```python
from build123d import *

# Parameters (mm, degrees)
CROQUIS4_R              = 4
SALIENTE_EXTRUIR1_DEPTH = 1.5
SALIENTE_EXTRUIR2_DEPTH = 6.9
SALIENTE_EXTRUIR3_DEPTH = 1.5
CORTAR_EXTRUIR1_DEPTH   = 1.5
REDONDEO1_R             = 3


with BuildPart() as part:
    # Croquis4 → Saliente-Extruir1 (new body)
    with BuildSketch(Plane.XY):
        with BuildLine():
            Line((-683.531695239, 333.374182683), (-683.531695239, 346.225865369))
            ThreePointArc((-683.531695239, 346.225865369), (-682.360122363, 349.054292493), (-679.531695239, 350.225865369))
            Line((-679.531695239, 350.225865369), (-666.680012553, 350.225865369))
            ThreePointArc((-666.680012553, 350.225865369), (-665.398822158, 349.872619004), (-664.479692443, 348.912706306))
            ThreePointArc((-664.479692443, 348.912706306), (-659.289054552, 341.941594121), (-652.317942367, 336.75095623))
            ThreePointArc((-652.317942367, 336.75095623), (-651.358029669, 335.831826514), (-651.004783304, 334.550636119))
            Line((-651.004783304, 334.550636119), (-667.856465989, 317.698953434))
            ThreePointArc((-667.856465989, 317.698953434), (-669.137656384, 318.052199798), (-670.0567861, 319.012112496))
            ThreePointArc((-670.0567861, 319.012112496), (-675.247423991, 325.983224681), (-682.218536176, 331.173862573))
            ThreePointArc((-682.218536176, 331.173862573), (-683.178448874, 332.092992288), (-683.531695239, 333.374182683))
        make_face()
        with Locations((-667.975346053, 334.669516182)):
            Circle(CROQUIS4_R, mode=Mode.SUBTRACT)
        with BuildLine():
            Line((-675.753520646, 345.629671291), (-673.632200302, 343.508350947))
            ThreePointArc((-673.632200302, 343.508350947), (-673.632200302, 340.326370432), (-676.814180817, 340.326370432))
            Line((-676.814180817, 340.326370432), (-678.935501161, 342.447690776))
            ThreePointArc((-678.935501161, 342.447690776), (-678.935501161, 345.629671291), (-675.753520646, 345.629671291))
        make_face(mode=Mode.SUBTRACT)
        with BuildLine():
            Line((-669.475346053, 344.419516182), (-669.475346053, 342.419516182))
            ThreePointArc((-669.475346053, 342.419516182), (-667.975346053, 340.919516182), (-666.475346053, 342.419516182))
            Line((-666.475346053, 342.419516182), (-666.475346053, 344.419516182))
            ThreePointArc((-666.475346053, 344.419516182), (-667.975346053, 345.919516182), (-669.475346053, 344.419516182))
        make_face(mode=Mode.SUBTRACT)
        with BuildLine():
            Line((-658.225346053, 336.169516182), (-660.225346053, 336.169516182))
            ThreePointArc((-660.225346053, 336.169516182), (-661.725346053, 334.669516182), (-660.225346053, 333.169516182))
            Line((-660.225346053, 333.169516182), (-658.225346053, 333.169516182))
            ThreePointArc((-658.225346053, 333.169516182), (-656.725346053, 334.669516182), (-658.225346053, 336.169516182))
        make_face(mode=Mode.SUBTRACT)
        with BuildLine():
            Line((-666.475346053, 324.919516182), (-666.475346053, 326.919516182))
            ThreePointArc((-666.475346053, 326.919516182), (-667.975346053, 328.419516182), (-669.475346053, 326.919516182))
            Line((-669.475346053, 326.919516182), (-669.475346053, 324.919516182))
            ThreePointArc((-669.475346053, 324.919516182), (-667.975346053, 323.419516182), (-666.475346053, 324.919516182))
        make_face(mode=Mode.SUBTRACT)
        with BuildLine():
            Line((-677.725346053, 333.169516182), (-675.725346053, 333.169516182))
            ThreePointArc((-675.725346053, 333.169516182), (-674.225346053, 334.669516182), (-675.725346053, 336.169516182))
            Line((-675.725346053, 336.169516182), (-677.725346053, 336.169516182))
            ThreePointArc((-677.725346053, 336.169516182), (-679.225346053, 334.669516182), (-677.725346053, 333.169516182))
        make_face(mode=Mode.SUBTRACT)
    extrude(amount=SALIENTE_EXTRUIR1_DEPTH)

    # Croquis5 → Saliente-Extruir2 (add)
    with BuildSketch(Plane(origin=(0, 0, 0), x_dir=(-1, 0, 0), z_dir=(0, 0, -1))):
        with BuildLine():
            ThreePointArc((670.0567861, 319.012112496), (669.137656384, 318.052199798), (667.856465989, 317.698953434))
            Line((667.856465989, 317.698953434), (669.532640967, 316.022778456))
            ThreePointArc((669.532640967, 316.022778456), (670.853714641, 316.842392616), (671.817042188, 318.062639746))
            ThreePointArc((671.817042188, 318.062639746), (676.661637554, 324.569011119), (683.168008926, 329.413606484))
            ThreePointArc((683.168008926, 329.413606484), (684.895851783, 331.068039972), (685.531695239, 333.374182683))
            Line((685.531695239, 333.374182683), (685.531695239, 346.225865369))
            ThreePointArc((685.531695239, 346.225865369), (683.774335926, 350.468506056), (679.531695239, 352.225865369))
            Line((679.531695239, 352.225865369), (666.680012553, 352.225865369))
            ThreePointArc((666.680012553, 352.225865369), (664.373869842, 351.590021913), (662.719436354, 349.862179056))
            ThreePointArc((662.719436354, 349.862179056), (657.874840989, 343.355807684), (651.368469617, 338.511212318))
            ThreePointArc((651.368469617, 338.511212318), (650.148222486, 337.547884771), (649.328608326, 336.226811097))
            Line((649.328608326, 336.226811097), (651.004783304, 334.550636119))
            ThreePointArc((651.004783304, 334.550636119), (651.358029669, 335.831826514), (652.317942367, 336.75095623))
            ThreePointArc((652.317942367, 336.75095623), (659.289054552, 341.941594121), (664.479692443, 348.912706306))
            ThreePointArc((664.479692443, 348.912706306), (665.398822158, 349.872619004), (666.680012553, 350.225865369))
            Line((666.680012553, 350.225865369), (679.531695239, 350.225865369))
            ThreePointArc((679.531695239, 350.225865369), (682.360122363, 349.054292493), (683.531695239, 346.225865369))
            Line((683.531695239, 346.225865369), (683.531695239, 333.374182683))
            ThreePointArc((683.531695239, 333.374182683), (683.178448874, 332.092992288), (682.218536176, 331.173862573))
            ThreePointArc((682.218536176, 331.173862573), (675.247423991, 325.983224681), (670.0567861, 319.012112496))
        make_face()
        with BuildLine():
            ThreePointArc((678.935501161, 342.447690776), (678.935501161, 345.629671291), (675.753520646, 345.629671291))
            Line((675.753520646, 345.629671291), (673.632200302, 343.508350947))
            ThreePointArc((673.632200302, 343.508350947), (673.632200302, 340.326370432), (676.814180817, 340.326370432))
            Line((676.814180817, 340.326370432), (678.935501161, 342.447690776))
        make_face()
    extrude(amount=-SALIENTE_EXTRUIR2_DEPTH)

    # Croquis6 → Saliente-Extruir3 (add)
    with BuildSketch(Plane.XY.offset(6.9)):
        with BuildLine():
            Line((-667.856465989, 319.198953434), (-667.100243806, 318.465261145))
            Line((-667.100243806, 318.465261145), (-669.532640967, 316.022778456))
            ThreePointArc((-669.532640967, 316.022778456), (-670.853714641, 316.842392616), (-671.817042188, 318.062639746))
            ThreePointArc((-671.817042188, 318.062639746), (-676.661637554, 324.569011119), (-683.168008926, 329.413606484))
            ThreePointArc((-683.168008926, 329.413606484), (-684.895851783, 331.068039972), (-685.531695239, 333.374182683))
            Line((-685.531695239, 333.374182683), (-685.531695239, 346.225865369))
            ThreePointArc((-685.531695239, 346.225865369), (-683.774335926, 350.468506056), (-679.531695239, 352.225865369))
            Line((-679.531695239, 352.225865369), (-666.680012553, 352.225865369))
            ThreePointArc((-666.680012553, 352.225865369), (-664.373869842, 351.590021913), (-662.719436354, 349.862179056))
            ThreePointArc((-662.719436354, 349.862179056), (-657.874840989, 343.355807684), (-651.368469617, 338.511212318))
            ThreePointArc((-651.368469617, 338.511212318), (-650.148222486, 337.547884771), (-649.328608326, 336.226811097))
            Line((-649.328608326, 336.226811097), (-651.765332209, 333.790087215))
            Line((-651.765332209, 333.790087215), (-652.503991007, 334.551428417))
            ThreePointArc((-652.503991007, 334.551428417), (-652.645289552, 335.063904575), (-653.029254632, 335.431556461))
            ThreePointArc((-653.029254632, 335.431556461), (-660.349095394, 340.881501273), (-665.799494351, 348.201003883))
            ThreePointArc((-665.799494351, 348.201003883), (-666.167146237, 348.584968962), (-666.679622395, 348.726267508))
            Line((-666.679622395, 348.726267508), (-679.53130508, 348.726267508))
            ThreePointArc((-679.53130508, 348.726267508), (-681.299072033, 347.994034461), (-682.03130508, 346.226267508))
            Line((-682.03130508, 346.226267508), (-682.03130508, 333.374584822))
            ThreePointArc((-682.03130508, 333.374584822), (-681.890006535, 332.862108664), (-681.506041455, 332.494456778))
            ThreePointArc((-681.506041455, 332.494456778), (-674.186373661, 327.044286992), (-668.736203875, 319.724619198))
            ThreePointArc((-668.736203875, 319.724619198), (-668.368791902, 319.340524583), (-667.856465989, 319.198953434))
        make_face()
    extrude(amount=SALIENTE_EXTRUIR3_DEPTH)

    # Croquis7 → Cortar-Extruir1 (cut)
    with BuildSketch(Plane.XY.offset(1.5)):
        with BuildLine():
            Line((-677.725346053, 330.669516182), (-666.305624647, 319.249794777))
            Line((-666.305624647, 319.249794777), (-652.555624647, 332.999794777))
            Line((-652.555624647, 332.999794777), (-663.975346053, 344.419516182))
            ThreePointArc((-663.975346053, 344.419516182), (-667.975346053, 348.419516182), (-671.975346053, 344.419516182))
            ThreePointArc((-671.975346053, 344.419516182), (-671.975346053, 338.669516182), (-677.725346053, 338.669516182))
            ThreePointArc((-677.725346053, 338.669516182), (-681.725346053, 334.669516182), (-677.725346053, 330.669516182))
        make_face()
    extrude(amount=-CORTAR_EXTRUIR1_DEPTH, mode=Mode.SUBTRACT)

    # Redondeo1
    redondeo1_edges = [part.edges().sort_by_distance(p)[0] for p in [
        (-677.725346053, 330.669516182, 0.75),
        (-677.725346053, 338.669516182, 0.75),
        (-671.975346053, 344.419516182, 0.75),
        (-663.975346053, 344.419516182, 0.75),
    ]]
    fillet(redondeo1_edges, radius=REDONDEO1_R)


solid = part.part
```
Could you check a few things on this model? Use its own coordinates, in mm. A direction names the side the tool comes from. Give positions to 0.01 mm unless a question says otherwise; leave off trailing zeros. Write each loop counter-clockwise with the first axis right and the second up, starting at its lowest first coordinate (ties: lowest second). Pieces come first, ordered by that corner, then holes. Notation, with made-up numbers: (-25.75, -10) - (-2.75, -10) arc R26 ccw to (-2.75, 28) - close; hole circle Ø11 at (18.25, 89.5). An arc over 180 degrees is marked (long way). One line per item, written item: value. Start each with the question number.
Item 1: Imagine slicing it at B-B, the plane x = -681. List the corners of the cut face in (y, z) for me.
Item 2: Imagine slicing it at C-C, the plane y = 343. List the corners of the cut face in (x, z) for me.
Item 3: Which directions (+Z, -Z, +X, -X, +Y, -Y) give clear straight access to the entire face, cutting with the end or side of a thin tool? Please do faces 1 (the face through (-669.15, 318.06, 4.16)), 2 (the face through (-673, 350.226, 4)), 3 (the face through (-671.72, 324.664, 0.76)), 4 (the face through (-657.82, 338.264, 0.76)), 5 (the face through (-660.26, 340.79, 7.64)).
Item 4: Imagine slicing it at D-D, the plane z = 7.75. List the corners of the cut face in (x, y) for me.
Item 5: If we mould it in two halves opening along Y, with no side actions, what happens to faces 6 (the face through (-665.38, 349.86, 4.16)), 7 (the face through (-673, 348.726, 8)), 8 (the face through (-681.61, 333.71, 0.76)), 9 (the face through (-674, 342, 0))? For each: +Y half, -Y half, draft (parallel to the pull), parting line (faces both ways), or undercut.
Item 6: I'm going to push flat-ended pins straight in: pin 1 (1 mm diameter, centred on y = 348.5, z = 5, fed in from -X); pin 2 (5.5 mm diameter, centred on x = -676, y = 344.5, fed in from +Z); pin 3 (16.5 mm diameter, centred on x = -672, y = 330, fed in from -Z); pin 4 (4.5 mm diameter, centred on y = 342.5, z = 5, fed in from +X). Where does each tip first touch, or does it pass through?
Item 7: Imagine slicing it at A-A, the plane z = 3. List the corners of the cut face in (x, y) for me.
Item 8: Please list where these lines run through material, in increasing order: line 1 (Z direction, x = -673.5, y = 324.5); line 2 (Y direction, x = -675, z = 3.5); line 3 (Y direction, x = -674, z = 5). Write a range as from..to.
Geometry says:
1. outline: (328.11, 0) - (332.37, 0) - (332.37, 1.5) - (330.48, 1.5) - (330.48, 6.9) - (332.22, 6.9) - (332.22, 8.4) - (328.11, 8.4) - close; (336.97, 0) - (352.04, 0) - (352.04, 8.4) - (348.25, 8.4) - (348.25, 6.9) - (349.95, 6.9) - (349.95, 1.5) - (336.97, 1.5) - close
2. outline: (-685.53, 0) - (-671.05, 0) - (-671.05, 1.5) - (-673.25, 1.5) - (-673.25, 6.9) - (-679.34, 6.9) - (-679.34, 1.5) - (-683.53, 1.5) - (-683.53, 6.9) - (-682.03, 6.9) - (-682.03, 8.4) - (-685.53, 8.4) - close; (-662.56, 0) - (-657.51, 0) - (-657.51, 8.4) - (-662.28, 8.4) - (-662.28, 6.9) - (-660.3, 6.9) - (-660.3, 1.5) - (-662.56, 1.5) - close
3. face 1: +X
3. face 2: none
3. face 3: +Z, -Z, +X
3. face 4: +Z, -Z, -Y
3. face 5: +Z, -Y
4. outline: (-685.53, 333.37) arc R4.5 ccw to (-683.17, 329.41) arc R28 cw to (-671.82, 318.06) arc R4.5 ccw to (-669.53, 316.02) - (-667.1, 318.47) - (-667.86, 319.2) arc R1 cw to (-668.74, 319.72) arc R31.5 ccw to (-681.51, 332.49) arc R1 cw to (-682.03, 333.37) - (-682.03, 346.23) arc R2.5 cw to (-679.53, 348.73) - (-666.68, 348.73) arc R1 cw to (-665.8, 348.2) arc R31.5 ccw to (-653.03, 335.43) arc R1 cw to (-652.5, 334.55) - (-651.77, 333.79) - (-649.33, 336.23) arc R4.5 ccw to (-651.37, 338.51) arc R28 cw to (-662.72, 349.86) arc R4.5 ccw to (-666.68, 352.23) - (-679.53, 352.23) arc R6 ccw to (-685.53, 346.23) - close
5. face 6: -Y half
5. face 7: undercut
5. face 8: undercut
5. face 9: draft
6. pin 1: x = -685.26
6. pin 2: z = 6.9
6. pin 3: z = 0
6. pin 4: x = -654.18
7. outline: (-685.53, 333.37) arc R4.5 ccw to (-683.17, 329.41) arc R28 cw to (-671.82, 318.06) arc R4.5 ccw to (-669.53, 316.02) - (-667.86, 317.7) arc R2.5 cw to (-670.06, 319.01) arc R30 ccw to (-682.22, 331.17) arc R2.5 cw to (-683.53, 333.37) - (-683.53, 346.23) arc R4 cw to (-679.53, 350.23) - (-666.68, 350.23) arc R2.5 cw to (-664.48, 348.91) arc R30 ccw to (-652.32, 336.75) arc R2.5 cw to (-651, 334.55) - (-649.33, 336.23) arc R4.5 ccw to (-651.37, 338.51) arc R28 cw to (-662.72, 349.86) arc R4.5 ccw to (-666.68, 352.23) - (-679.53, 352.23) arc R6 ccw to (-685.53, 346.23) - close; (-678.94, 342.45) - (-676.81, 340.33) arc R2.25 ccw to (-673.63, 343.51) - (-675.75, 345.63) arc R2.25 ccw to start
8. line 1: 0..1.5, 6.9..8.4
8. line 2: 322.75..325.73, 339.68..344.88, 350.23..352.23
8. line 3: 321.49..324.66, 340.03..343.88, 350.23..352.23
